Part model, mm, in its own coordinate system. Round coordinates to 2 decimals unless told otherwise and drop trailing zeros. Order: outer loops, then holes, each group sorted by start corner. A loop starts at its lowest first (then second) coordinate and runs counter-clockwise, first axis right, second up. Notation, with made-up numbers: (23, -30) - (78, -30) arc R8 cw to (78, -22) - close; hole circle Ø1 at (-39, -2.5). An arc over 180 degrees is marked (long way). Return JSON: item names as keys, results as strings. Group by question number.
Item 1: Saw through at B-B on z = -16.25. List the corners of the cut face in (x, y).
Item 2: Saw through at C-C on y = 3. List the corners of the cut face in (x, z), and give its area (3 significant figures).
Item 3: Two-plate mould, pull along X, no slides. Class faces 1 (the face through (28.016, 3.479, 17.771)), 2 (the face through (50, 2, 0)), 3 (the face through (14, 5, 0)): released by +X, released by -X, zero draft, split by the parting line, or undercut.
Item 4: Drop a flat-ended pin along its axis: pin 1 (2 mm diameter, centred on y = 2.5, z = 1.5, fed in from -X). Give the stop position or say it passes through.
Item 5: Saw through at D-D on z = 10.5. List the corners of the cut face in (x, y).
Item 6: Saw through at A-A on x = 30. List the corners of the cut face in (y, z).
Item 7: Probe probe 1 along Z at (x, y) = (30, 4.2); probe 2 along X at (y, z) = (3.6, 17); probe 3 along X at (y, z) = (4.1, 16.25). List the from-to ranges inside material, lowest first.
```python
from build123d import *

# Parameters (mm, degrees)
BOSS_EXTRUDE1_DEPTH     = 5
SKETCH2_R               = 2.5
CUT_EXTRUDE1_DEPTH      = 6
CUT_EXTRUDE1_DEPTH_BACK = 1
CHAMFER1_SIZE           = 2


with BuildPart() as part:
    # Sketch1 → Boss-Extrude1 (new body)
    with BuildSketch(Plane(origin=(0, 0, 0), x_dir=(1, 0, 0), z_dir=(0, 1, 0))):
        with BuildLine():
            Line((0, 22.5), (50, 22.5))
            Line((50, 22.5), (50, -22.5))
            Line((50, -22.5), (0, -22.5))
            ThreePointArc((0, -22.5), (-22.5, 0), (0, 22.5))
        make_face()
    extrude(amount=BOSS_EXTRUDE1_DEPTH)

    # Sketch2 → Cut-Extrude1 (cut, two sides)
    with BuildSketch(Plane(origin=(0, 0, 0), x_dir=(1, 0, 0), z_dir=(0, 1, 0))) as cut_extrude1_sk:
        with Locations((30, 16.25)):
            Circle(SKETCH2_R)
        with Locations((30, -16.25)):
            Circle(SKETCH2_R)
    extrude(amount=CUT_EXTRUDE1_DEPTH, mode=Mode.SUBTRACT)
    extrude(cut_extrude1_sk.sketch, amount=-CUT_EXTRUDE1_DEPTH_BACK, mode=Mode.SUBTRACT)

    # Chamfer1
    chamfer1_edges = [part.edges().sort_by_distance(p)[0] for p in [
        (27.5, 0, -16.25),
        (27.5, 0, 16.25),
    ]]
    chamfer(chamfer1_edges, length=CHAMFER1_SIZE)


solid = part.part
```
Filled in:
{
 "1": {"outline": "(-15.56, 0) - (25.5, 0) - (27.5, 2) - (27.5, 5) - (-15.56, 5) - close; (32.5, 2) - (34.5, 0) - (50, 0) - (50, 5) - (32.5, 5) - close"},
 "2": {"outline": "(0, -22.5) - (50, -22.5) - (50, 22.5) - (0, 22.5) arc R22.5 ccw to start; hole circle Ø5 at (30, -16.25); hole circle Ø5 at (30, 16.25)", "area": "3,010 mm^2"},
 "3": {"face 1": "undercut", "face 2": "released by +X", "face 3": "zero draft"},
 "4": {"pin 1": "stops at x = -22.49"},
 "5": {"outline": "(-19.9, 0) - (50, 0) - (50, 5) - (-19.9, 5) - close"},
 "6": {"outline": "(0, -22.5) - (5, -22.5) - (5, -18.75) - (2, -18.75) - (0, -20.75) - close; (0, -11.75) - (2, -13.75) - (5, -13.75) - (5, 13.75) - (2, 13.75) - (0, 11.75) - close; (0, 20.75) - (2, 18.75) - (5, 18.75) - (5, 22.5) - (0, 22.5) - close"},
 "7": {"probe 1": "z = -22.5 to -18.75, -13.75 to 13.75, 18.75 to 22.5", "probe 2": "x = -14.74 to 27.62, 32.38 to 50", "probe 3": "x = -15.56 to 27.5, 32.5 to 50"}
}
